```python
from build123d import *

# Parameters (mm, degrees)
SKETCH_1_W                = 101
SKETCH_1_H                = 26.5
EXTRUDE_1_DEPTH           = 2.5
SKETCH_2_W                = 101
SKETCH_2_H                = 26.5
SKETCH_2_W_2              = 96
SKETCH_2_H_2              = 21.5
EXTRUDE_2_DEPTH           = 21.5
SKETCH_3_W                = 4
SKETCH_3_H                = 4
EXTRUDE_3_DEPTH           = 19
SKETCH_5_R                = 1
CUT_EXTRUDE_1_DEPTH       = 12
SKETCH_6_W                = 45
SKETCH_6_H                = 13
CUT_EXTRUDE_2_DEPTH       = 1.5
SKETCH_7_W                = 4
SKETCH_7_H                = 13
CUT_EXTRUDE_3_DEPTH       = 1.5
SKETCH_8_W                = 97
SKETCH_8_H                = 22.5
CUT_EXTRUDE_4_DEPTH       = 2.5
CUT_EXTRUDE_5_REACH       = 109.141
SKETCH_9_W                = 10
SKETCH_9_H                = 2
SKETCH_9_W_2              = 3
SKETCH_9_H_2              = 1.5
CHAMFER_1_SIZE            = 2
CUT_EXTRUDE_6_REACH       = 109.141
SKETCH_11_W               = 3
SKETCH_11_H               = 1.5
CUT_EXTRUDE_7_REACH       = 109.141
SKETCH_12_W               = 3
SKETCH_12_H               = 3
SKETCH_14_W               = 4
SKETCH_14_H               = 5.5
SKETCH_14_W_2             = 3
SKETCH_14_H_2             = 3
EXTRUDE_4_DEPTH           = 5
CUT_EXTRUDE_8_REACH       = 109.141
SKETCH_13_W               = 3
SKETCH_13_H               = 3
SKETCH_15_W               = 4
SKETCH_15_H               = 5.5
EXTRUDE_5_DEPTH           = 1.5
SKETCH_16_W               = 19
SKETCH_16_H               = 21.5
EXTRUDE_6_DEPTH           = 1
CUT_EXTRUDE_START         = -2.5
CUT_EXTRUDE_9_OUTLINE_W   = 17
CUT_EXTRUDE_9_OUTLINE_H   = 1
CUT_EXTRUDE_9_OUTLINE_W_2 = 24
CUT_EXTRUDE_9_DEPTH       = 2.5


# Read off the part's stored shape, not the designer's step: 切除-拉伸9
with BuildPart() as part:
    # 草图1 → 凸台-拉伸1 (new body)
    with BuildSketch(Plane.XY):
        with Locations((50.5, 13.25)):
            Rectangle(SKETCH_1_W, SKETCH_1_H)
    extrude(amount=EXTRUDE_1_DEPTH)

    # 草图2 → 凸台-拉伸2 (add)
    with BuildSketch(Plane.XY.offset(2.5)):
        with Locations((50.5, 13.25)):
            Rectangle(SKETCH_2_W, SKETCH_2_H)
        with Locations((50.5, 13.25)):
            Rectangle(SKETCH_2_W_2, SKETCH_2_H_2, mode=Mode.SUBTRACT)
    extrude(amount=EXTRUDE_2_DEPTH)

    # 草图3 → 凸台-拉伸3 (add)
    with BuildSketch(Plane.XY.offset(2.5)):
        with Locations((4.5, 22)):
            Rectangle(SKETCH_3_W, SKETCH_3_H)
        with Locations((4.5, 4.5)):
            Rectangle(SKETCH_3_W, SKETCH_3_H)
        Polygon((98.5, 24), (95.195835911, 24), (95.195835911, 20), (95.195835911, 6.5), (95.195835911, 2.5), (98.5, 2.5), (98.5, 8.754439991), (98.5, 17.745560009), align=None)
    extrude(amount=EXTRUDE_3_DEPTH)

    # 草图5 → 切除-拉伸1 (cut)
    with BuildSketch(Plane.XY.offset(21.5)):
        with Locations((4.5, 22)):
            Circle(SKETCH_5_R)
        with Locations((4.5, 4.5)):
            Circle(SKETCH_5_R)
        with Locations((96.5, 22)):
            Circle(SKETCH_5_R)
        with Locations((96.5, 4.5)):
            Circle(SKETCH_5_R)
    extrude(amount=-CUT_EXTRUDE_1_DEPTH, mode=Mode.SUBTRACT)

    # 草图6 → 切除-拉伸2 (cut)
    with BuildSketch(Plane.XZ):
        with Locations((32.5, 12.5)):
            Rectangle(SKETCH_6_W, SKETCH_6_H)
    extrude(amount=-CUT_EXTRUDE_2_DEPTH, mode=Mode.SUBTRACT)

    # 草图7 → 切除-拉伸3 (cut)
    with BuildSketch(Plane.XZ.offset(-1.5)):
        with Locations((12, 12.5)):
            Rectangle(SKETCH_7_W, SKETCH_7_H)
    extrude(amount=-CUT_EXTRUDE_3_DEPTH, mode=Mode.SUBTRACT)

    # 草图8 → 切除-拉伸4 (cut)
    with BuildSketch(Plane.XY.offset(24)):
        with Locations((50.5, 13.25)):
            Rectangle(SKETCH_8_W, SKETCH_8_H)
    extrude(amount=-CUT_EXTRUDE_4_DEPTH, mode=Mode.SUBTRACT)

    # 草图9 → 切除-拉伸5 (cut, up to next)
    with BuildSketch(Plane.XZ, mode=Mode.PRIVATE) as cut_extrude_5_sk1:
        with Locations((11.25, 23)):
            Rectangle(SKETCH_9_W, SKETCH_9_H)
    cut_extrude_5_tool1 = extrude(cut_extrude_5_sk1.sketch, amount=-CUT_EXTRUDE_5_REACH, mode=Mode.PRIVATE) & part.part
    # 草图9 → 切除-拉伸5 (cut, up to next)
    with BuildSketch(Plane.XZ, mode=Mode.PRIVATE) as cut_extrude_5_sk2:
        with Locations((19.75, 23.25)):
            Rectangle(SKETCH_9_W_2, SKETCH_9_H_2)
    cut_extrude_5_tool2 = extrude(cut_extrude_5_sk2.sketch, amount=-CUT_EXTRUDE_5_REACH, mode=Mode.PRIVATE) & part.part
    # 草图9 → 切除-拉伸5 (cut, up to next)
    with BuildSketch(Plane.XZ, mode=Mode.PRIVATE) as cut_extrude_5_sk3:
        with Locations((27.75, 23.25)):
            Rectangle(SKETCH_9_W_2, SKETCH_9_H_2)
    cut_extrude_5_tool3 = extrude(cut_extrude_5_sk3.sketch, amount=-CUT_EXTRUDE_5_REACH, mode=Mode.PRIVATE) & part.part
    # 草图9 → 切除-拉伸5 (cut, up to next)
    with BuildSketch(Plane.XZ, mode=Mode.PRIVATE) as cut_extrude_5_sk4:
        with Locations((35.75, 23.25)):
            Rectangle(SKETCH_9_W_2, SKETCH_9_H_2)
    cut_extrude_5_tool4 = extrude(cut_extrude_5_sk4.sketch, amount=-CUT_EXTRUDE_5_REACH, mode=Mode.PRIVATE) & part.part
    add(cut_extrude_5_tool1.solids().sort_by_distance((11.25, 0, 23))[0], mode=Mode.SUBTRACT)
    add(cut_extrude_5_tool2.solids().sort_by_distance((19.75, 0, 23.25))[0], mode=Mode.SUBTRACT)
    add(cut_extrude_5_tool3.solids().sort_by_distance((27.75, 0, 23.25))[0], mode=Mode.SUBTRACT)
    add(cut_extrude_5_tool4.solids().sort_by_distance((35.75, 0, 23.25))[0], mode=Mode.SUBTRACT)

    # 倒角1
    chamfer_1_edges = [part.edges().sort_by_distance(p)[0] for p in [
        (16.25, 0, 23),
        (11.25, 0, 22),
        (6.25, 0, 23),
    ]]
    chamfer(chamfer_1_edges, length=CHAMFER_1_SIZE - 0.0001)  # a hair under: the kernel refuses the full size

    # 草图11 → 切除-拉伸6 (cut, up to next)
    with BuildSketch(Plane(origin=(0, 26.5, 0), x_dir=(1, 0, 0), z_dir=(0, 1, 0)), mode=Mode.PRIVATE) as cut_extrude_6_sk1:
        with Locations((27, -23.25)):
            Rectangle(SKETCH_11_W, SKETCH_11_H)
    cut_extrude_6_tool1 = extrude(cut_extrude_6_sk1.sketch, amount=-CUT_EXTRUDE_6_REACH, mode=Mode.PRIVATE) & part.part
    # 草图11 → 切除-拉伸6 (cut, up to next)
    with BuildSketch(Plane(origin=(0, 26.5, 0), x_dir=(1, 0, 0), z_dir=(0, 1, 0)), mode=Mode.PRIVATE) as cut_extrude_6_sk2:
        with Locations((35, -23.25)):
            Rectangle(SKETCH_11_W, SKETCH_11_H)
    cut_extrude_6_tool2 = extrude(cut_extrude_6_sk2.sketch, amount=-CUT_EXTRUDE_6_REACH, mode=Mode.PRIVATE) & part.part
    add(cut_extrude_6_tool1.solids().sort_by_distance((27, 26.5, 23.25))[0], mode=Mode.SUBTRACT)
    add(cut_extrude_6_tool2.solids().sort_by_distance((35, 26.5, 23.25))[0], mode=Mode.SUBTRACT)

    # 草图12 → 切除-拉伸7 (cut, up to next)
    with BuildSketch(Plane(origin=(0, 0, 0), x_dir=(-1, 0, 0), z_dir=(0, 0, -1)), mode=Mode.PRIVATE) as cut_extrude_7_sk1:
        with Locations((-4.5, 17)):
            Rectangle(SKETCH_12_W, SKETCH_12_H)
    cut_extrude_7_tool1 = extrude(cut_extrude_7_sk1.sketch, amount=-CUT_EXTRUDE_7_REACH, mode=Mode.PRIVATE) & part.part
    add(cut_extrude_7_tool1.solids().sort_by_distance((4.5, 17, 0))[0], mode=Mode.SUBTRACT)

    # 草图14 → 凸台-拉伸4 (add)
    with BuildSketch(Plane.XY.offset(2.5)):
        with Locations((4.5, 17.25)):
            Rectangle(SKETCH_14_W, SKETCH_14_H)
        with Locations((4.5, 17)):
            Rectangle(SKETCH_14_W_2, SKETCH_14_H_2, mode=Mode.SUBTRACT)
    extrude(amount=EXTRUDE_4_DEPTH)

    # 草图13 → 切除-拉伸8 (cut, up to next)
    with BuildSketch(Plane.ZY, mode=Mode.PRIVATE) as cut_extrude_8_sk1:
        with Locations((4.5, 17)):
            Rectangle(SKETCH_13_W, SKETCH_13_H)
    cut_extrude_8_tool1 = extrude(cut_extrude_8_sk1.sketch, amount=-CUT_EXTRUDE_8_REACH, mode=Mode.PRIVATE) & part.part
    add(cut_extrude_8_tool1.solids().sort_by_distance((0, 17, 4.5))[0], mode=Mode.SUBTRACT)

    # 草图15 → 凸台-拉伸5 (add)
    with BuildSketch(Plane.XY.offset(7.5)):
        with Locations((4.5, 17.25)):
            Rectangle(SKETCH_15_W, SKETCH_15_H)
    extrude(amount=-EXTRUDE_5_DEPTH)

    # 草图16 → 凸台-拉伸6 (add)
    with BuildSketch(Plane.ZY.offset(-95.195835911)):
        with Locations((12, 13.25)):
            Rectangle(SKETCH_16_W, SKETCH_16_H)
    extrude(amount=EXTRUDE_6_DEPTH)

    # 切除-拉伸9 outline → 切除-拉伸9 (cut)
    with BuildSketch(Plane.XY.offset(24).offset(CUT_EXTRUDE_START)):
        with Locations((31, 25)):
            Rectangle(CUT_EXTRUDE_9_OUTLINE_W, CUT_EXTRUDE_9_OUTLINE_H)
        with Locations((28.25, 1.5)):
            Rectangle(CUT_EXTRUDE_9_OUTLINE_W_2, CUT_EXTRUDE_9_OUTLINE_H)
    extrude(amount=CUT_EXTRUDE_9_DEPTH, mode=Mode.SUBTRACT)


solid = part.part
```
Can you work these out from the model? Positions are in its coordinate system, mm. A direction names the side the tool comes from. Round coordinates to 2 decimals unless told otherwise and drop trailing zeros. Loops run counter-clockwise (first coordinate to the right, second up) from the corner with the lowest first, then second, coordinate; pieces in that order, holes last. Notation, with made-up numbers: M 63,-14.75 L 96,-14.75 A25 cw 96,15.25 Z; hole C 70.5,-38.75 d4. An arc over 180 degrees is marked long. Answer in a Markdown table with one row per item.
1. If we section it at B-B, the plane y = 4.5: Please give me the cut outline in (x, z), plus the area to 3 significant figures.
Established:
| item | result |
|---|---|
| outline | M 0,0 L 101,0 L 101,24 L 99,24 L 99,21.5 L 97.5,21.5 L 97.5,9.5 L 95.5,9.5 L 95.5,21.5 L 94.2,21.5 L 94.2,2.5 L 6.5,2.5 L 6.5,21.5 L 5.5,21.5 L 5.5,9.5 L 3.5,9.5 L 3.5,21.5 L 2,21.5 L 2,24 L 0,24 Z |
| area | 467 mm² |
2. If we section it at D-D, the plane x = 59: Please give me the cut outline in (y, z), plus the area to 3 significant figures.
Established:
| item | result |
|---|---|
| outline | M 0,0 L 26.5,0 L 26.5,24 L 24.5,24 L 24.5,21.5 L 24,21.5 L 24,2.5 L 2.5,2.5 L 2.5,21.5 L 2,21.5 L 2,24 L 0,24 Z |
| area | 171 mm² |
3. Please list where these lines run through material, in increasing order: line 1 (Y direction, x = 4.5, z = 16.5); line 2 (Y direction, x = 96.5, z = 17); line 3 (X direction, y = 8, z = 5.75). Write a range as from..to.
Established:
| item | result |
|---|---|
| line 1 | 0..3.5, 5.5..6.5, 20..21, 23..26.5 |
| line 2 | 0..3.5, 5.5..21, 23..26.5 |
| line 3 | 0..2.5, 94.2..101 |
4. I'm going to push flat-ended pins straight in: pin 1 Ø1.6 at (x, y) = (96.5, 4.5) entering from +Z; pin 2 Ø1.5 at (x, y) = (81.5, 18) entering from +Z. Where does each tip first touch, or does it pass through?
Established:
| item | result |
|---|---|
| pin 1 | z = 9.5 |
| pin 2 | z = 2.5 |
5. If we section it at C-C, the plane z = 16.25: Please give me the cut outline in (x, y), plus the area to 3 significant figures.
Established:
| item | result |
|---|---|
| outline | M 0,0 L 10,0 L 10,2.5 L 6.5,2.5 L 6.5,6.5 L 2.5,6.5 L 2.5,20 L 6.5,20 L 6.5,24 L 94.2,24 L 94.2,2.5 L 14,2.5 L 14,1.5 L 55,1.5 L 55,0 L 101,0 L 101,26.5 L 0,26.5 Z; hole C 4.5,4.5 d2; hole C 4.5,22 d2; hole C 96.5,4.5 d2; hole C 96.5,22 d2 |
| area | 653 mm² |
6. Thinking about a two-plate mould opening in Z: for faces 1 (the face through (4, 15.5, 4)), 2 (the face through (69, 24.5, 23)), 3 (the face through (96, 22, 9.5)), which applies, pulls with the +Z half, pulls with the -Z half, needs draft (parallel to the pull), parting line crosses it, or undercut?
Established:
| item | result |
|---|---|
| face 1 | undercut |
| face 2 | needs draft |
| face 3 | pulls with the +Z half |
7. On a 3-axis mill with a long thin cutter (end or side, diameter ignored), from which of +Z, -Z, +X, -X, +Y, -Y can I reach the whole of each face in a straight line? I mean faces 4 (the face through (95.5, 4.5, 15.6)), 5 (the face through (4, 18.5, 4)), 6 (the face through (73, 25, 24)), 7 (the face through (1, 17, 3)). Say none if no direction works.
Established:
| item | result |
|---|---|
| face 4 | +Z |
| face 5 | none |
| face 6 | +Z, +X, -X, +Y, -Y |
| face 7 | -X |
